```python
from build123d import *

# Parameters (mm, degrees)
BASE_FLANGE1_START             = -2
BASE_FLANGE1_DEPTH             = 2
EDGE_FLANGE1_STRIP_W           = 9.4732
EDGE_FLANGE1_STRIP_H           = 2
EDGE_FLANGE1_STRIP_CUT_DEPTH   = 254
EDGE_FLANGE1_STRIP_2_W         = 9.4732
EDGE_FLANGE1_STRIP_2_H         = 2
EDGE_FLANGE1_STRIP_CUT_2_DEPTH = 254
EDGE_FLANGE1_DEPTH             = 254
EDGE_FLANGE1_BEND_DEPTH        = 254
EDGE_FLANGE2_STRIP_W           = 9.4732
EDGE_FLANGE2_STRIP_H           = 2
EDGE_FLANGE2_STRIP_CUT_DEPTH   = 220
EDGE_FLANGE2_DEPTH             = 220
SKETCH15_R                     = 2
SKETCH15_R_2                   = 9.75
CUT_EXTRUDE1_DEPTH             = 178.482393493
SKETCH16_W                     = 25
SKETCH16_H                     = 7
SKETCH16_R                     = 2
CUT_EXTRUDE2_DEPTH             = 261.384331326


# Read off the part's stored shape, not the designer's step: Base-Flange1
# Sheet-metal steps are written as plain solids
with BuildPart() as part:
    # Base-Flange1 outline → Base-Flange1 (new body)
    with BuildSketch(Plane(origin=(0, 0, 0), x_dir=(1, 0, 0), z_dir=(0, 1, 0)).offset(BASE_FLANGE1_START)):
        Polygon((105, 126), (110, 126), (110, 130), (-110, 130), (-110, 126), (-105, 126), (-105, 124), (-110, 124), (-110, -130), (110, -130), (110, 124), (105, 124), align=None)
    extrude(amount=BASE_FLANGE1_DEPTH)

    # Edge-Flange1 strip (across the edge) → Edge-Flange1 strip cut (cut)
    with BuildSketch(Plane(origin=(-110, 0, -124), x_dir=(1, 0, 0), z_dir=(0, 0, 1))):
        with Locations((-2, -1)):
            Rectangle(EDGE_FLANGE1_STRIP_W, EDGE_FLANGE1_STRIP_H)
    extrude(amount=EDGE_FLANGE1_STRIP_CUT_DEPTH, mode=Mode.SUBTRACT)

    # Edge-Flange1 strip 2 (across the edge) → Edge-Flange1 strip cut 2 (cut)
    with BuildSketch(Plane(origin=(110, 0, 130), x_dir=(-1, 0, 0), z_dir=(0, 0, -1))):
        with Locations((-2, -1)):
            Rectangle(EDGE_FLANGE1_STRIP_2_W, EDGE_FLANGE1_STRIP_2_H)
    extrude(amount=EDGE_FLANGE1_STRIP_CUT_2_DEPTH, mode=Mode.SUBTRACT)

    # Edge-Flange1 section (across the edge) → Edge-Flange1 (add)
    with BuildSketch(Plane(origin=(-110, 0, -124), x_dir=(1, 0, 0), z_dir=(0, 0, 1))):
        with BuildLine():
            Line((0, 0.7366), (0, 50))
            Line((0, 50), (2, 50))
            Line((2, 50), (2, 0.7366))
            ThreePointArc((2, 0.7366), (2.215745145, 0.215745145), (2.7366, 0))
            Line((2.7366, 0), (2.7366, -2))
            ThreePointArc((2.7366, -2), (0.801531583, -1.198468417), (0, 0.7366))
        make_face()
    extrude(amount=EDGE_FLANGE1_DEPTH)

    # Edge-Flange1 section 2 (across the edge) → Edge-Flange1 bend (add)
    with BuildSketch(Plane(origin=(110, 0, 130), x_dir=(-1, 0, 0), z_dir=(0, 0, -1))):
        with BuildLine():
            Line((0, 0.7366), (0, 50))
            Line((0, 50), (2, 50))
            Line((2, 50), (2, 0.7366))
            ThreePointArc((2, 0.7366), (2.215745145, 0.215745145), (2.7366, 0))
            Line((2.7366, 0), (2.7366, -2))
            ThreePointArc((2.7366, -2), (0.801531583, -1.198468417), (0, 0.7366))
        make_face()
    extrude(amount=EDGE_FLANGE1_BEND_DEPTH)

    # Edge-Flange2 strip (across the edge) → Edge-Flange2 strip cut (cut)
    with BuildSketch(Plane(origin=(110, 0, -130), x_dir=(0, 0, 1), z_dir=(-1, 0, 0))):
        with Locations((-2, -1)):
            Rectangle(EDGE_FLANGE2_STRIP_W, EDGE_FLANGE2_STRIP_H)
    extrude(amount=EDGE_FLANGE2_STRIP_CUT_DEPTH, mode=Mode.SUBTRACT)

    # Edge-Flange2 section (across the edge) → Edge-Flange2 (add)
    with BuildSketch(Plane(origin=(110, 0, -130), x_dir=(0, 0, 1), z_dir=(-1, 0, 0))):
        with BuildLine():
            Line((0, 0.7366), (0, 3))
            Line((0, 3), (2, 3))
            Line((2, 3), (2, 0.7366))
            ThreePointArc((2, 0.7366), (2.215745145, 0.215745145), (2.7366, 0))
            Line((2.7366, 0), (2.7366, -2))
            ThreePointArc((2.7366, -2), (0.801531583, -1.198468417), (0, 0.7366))
        make_face()
    extrude(amount=EDGE_FLANGE2_DEPTH)

    # Sketch15 → Cut-Extrude1 (cut, through all)
    with BuildSketch(Plane(origin=(0, 0, 0), x_dir=(1, 0, 0), z_dir=(0, 1, 0))):
        Polygon((-85, -15), (-85, 105), (85, 105), (85, -15), (65, -45), (-65, -45), align=None)
        with Locations(Location((82, -107, 0), (0, 0, 270))):
            Circle(SKETCH15_R)
        with Locations(Location((67.5, -92.5, 0), (0, 0, 270))):
            Circle(SKETCH15_R)
        with Locations(Location((53, -107, 0), (0, 0, 270))):
            Circle(SKETCH15_R)
        with Locations(Location((67.5, -121.5, 0), (0, 0, 270))):
            Circle(SKETCH15_R)
        with Locations(Location((67.5, -107, 0), (0, 0, 270))):
            Circle(SKETCH15_R_2)
        with BuildLine():
            ThreePointArc((0, -85.5), (-10.5, -96), (0, -106.5))
            Line((0, -106.5), (0, -85.5))
        make_face()
        with BuildLine():
            Line((0, -85.5), (0, -106.5))
            ThreePointArc((0, -106.5), (7.424621202, -103.424621202), (10.5, -96))
            ThreePointArc((10.5, -96), (7.424621202, -88.575378798), (0, -85.5))
        make_face()
        with BuildLine():
            Line((0, -122), (0, -130))
            Line((0, -130), (65, -130))
            ThreePointArc((65, -130), (62.885553403, -129.850222745), (60.81333294, -129.403882079))
            Line((60.81333294, -129.403882079), (37.391782876, -122.596117921))
            ThreePointArc((37.391782876, -122.596117921), (35.319562413, -122.149777255), (33.205115817, -122))
            Line((33.205115817, -122), (0, -122))
        make_face()
        with BuildLine():
            Line((-65, -130), (0, -130))
            Line((0, -130), (0, -122))
            Line((0, -122), (-33.205115817, -122))
            ThreePointArc((-33.205115817, -122), (-35.319562413, -122.149777255), (-37.391782876, -122.596117921))
            Line((-37.391782876, -122.596117921), (-60.81333294, -129.403882079))
            ThreePointArc((-60.81333294, -129.403882079), (-62.885553403, -129.850222745), (-65, -130))
        make_face()
        with Locations(Location((16, -96, 0), (0, 0, 270))):
            Circle(SKETCH15_R)
        with Locations(Location((-16, -96, 0), (0, 0, 270))):
            Circle(SKETCH15_R)
        with Locations(Location((-67.5, -107, 0), (0, 0, 270))):
            Circle(SKETCH15_R_2)
        with Locations(Location((-53, -107, 0), (0, 0, 270))):
            Circle(SKETCH15_R)
        with Locations(Location((-67.5, -92.5, 0), (0, 0, 270))):
            Circle(SKETCH15_R)
        with Locations(Location((-67.5, -121.5, 0), (0, 0, 270))):
            Circle(SKETCH15_R)
        with Locations(Location((-82, -107, 0), (0, 0, 270))):
            Circle(SKETCH15_R)
        with Locations(Location((-90, -45, 0), (0, 0, 270))):
            Circle(SKETCH15_R)
        with Locations(Location((90, 115, 0), (0, 0, 90))):
            Circle(SKETCH15_R)
        with Locations(Location((90, -45, 0), (0, 0, 90))):
            Circle(SKETCH15_R)
        with Locations(Location((-90, 115, 0), (0, 0, 270))):
            Circle(SKETCH15_R)
    extrude(amount=-CUT_EXTRUDE1_DEPTH, mode=Mode.SUBTRACT)

    # Sketch16 → Cut-Extrude2 (cut, through all)
    with BuildSketch(Plane.ZY.offset(110)):
        with BuildLine():
            ThreePointArc((-124, 10.7366), (-122.535533906, 14.272133906), (-119, 15.7366))
            Line((-119, 15.7366), (53.501367481, 15.7366))
            ThreePointArc((53.501367481, 15.7366), (59.500667262, 17.736074884), (63.100877196, 22.934919573))
            Line((63.100877196, 22.934919573), (68.899122804, 42.801680427))
            ThreePointArc((68.899122804, 42.801680427), (72.499332738, 48.000525116), (78.498632519, 50))
            Line((78.498632519, 50), (-124, 50))
            Line((-124, 50), (-124, 10.7366))
        make_face()
        with Locations((38.5, 8.2366)):
            Rectangle(SKETCH16_W, SKETCH16_H)
        with Locations((3.5, 8.2366)):
            Rectangle(SKETCH16_W, SKETCH16_H)
        with Locations((-31.5, 8.2366)):
            Rectangle(SKETCH16_W, SKETCH16_H)
        with Locations((-66.5, 8.2366)):
            Rectangle(SKETCH16_W, SKETCH16_H)
        with Locations((-101.5, 8.2366)):
            Rectangle(SKETCH16_W, SKETCH16_H)
        with Locations(Location((86, 43, 0), (0, 0, 270))):
            Circle(SKETCH16_R)
        with Locations(Location((86, 23, 0), (0, 0, 270))):
            Circle(SKETCH16_R)
        with Locations(Location((119, 43, 0), (0, 0, 270))):
            Circle(SKETCH16_R)
        with Locations(Location((119, 23, 0), (0, 0, 270))):
            Circle(SKETCH16_R)
    extrude(amount=-CUT_EXTRUDE2_DEPTH, mode=Mode.SUBTRACT)


solid = part.part
```
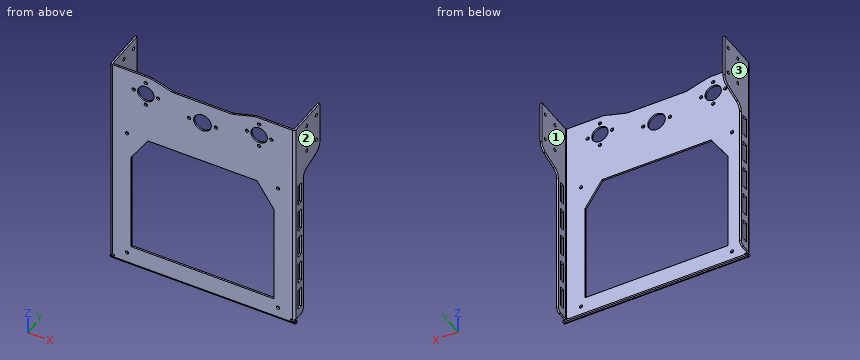
Geometry check sheet. Reference: the model listing, model coordinates, mm. Face numbers are marked on the shaded views. Coordinates: 2 decimals unless noted, no trailing zeros. Order: outer loops, then holes, each group sorted by start corner. A loop starts at its lowest first (then second) coordinate and runs counter-clockwise, first axis right, second up.
Item 1: Mould release check, pull along X, two halves, no side actions. Record for the marked faces 1, 2 and 3: released by +X, released by -X, zero draft, split by the parting line, or undercut.
Item 2: Scan lines: line 1 along Z through (x, y) = (-108.4, 23); line 2 along Z through (x, y) = (-109.3, 43); line 3 along X through (y, z) = (5, -17.5). Record each from-to range of solid material in increasing order.
Item 3: Section check A-A (z = -27). Enter the section's corners in (x, y), plus the area to 3 significant figures.
Item 4: Section check C-C (z = 20.5). Enter the section's corners in (x, y), plus the area to 3 significant figures.
Item 5: Section check B-B (y = 7.5). Count the separate pieces of the cut face and the enclosed holes in it, plus the area to 3 significant figures.
Item 6: Depth check by flat-ended pin: pin 1 (3.5 mm diameter, centred on x = 82, z = 107, fed in from -Y); pin 2 (1.6 mm diameter, centred on y = -1, z = -124.5, fed in from +X); pin 3 (2 mm diameter, centred on x = 19.5, y = -1, fed in from +Z); pin 4 (2 mm diameter, centred on x = -109, z = 9.5, fed in from -Y). Enter the tip coordinate at first touch or a pass-through.
Check sheet entries:
1. face 1: undercut
1. face 2: released by +X
1. face 3: released by -X
2. line 1: z = 63.12 to 84, 88 to 117, 121 to 130
2. line 2: z = 68.96 to 84, 88 to 117, 121 to 130
2. line 3: x = -110 to -108, 108 to 110
3. outline: (-110, 0.74) arc R2.74 ccw to (-107.26, -2) - (-85, -2) - (-85, 0) - (-107.26, 0) arc R0.74 cw to (-108, 0.74) - (-108, 4.74) - (-110, 4.74) - close; (-110, 11.74) - (-108, 11.74) - (-108, 15.74) - (-110, 15.74) - close; (85, -2) - (107.26, -2) arc R2.74 ccw to (110, 0.74) - (110, 4.74) - (108, 4.74) - (108, 0.74) arc R0.74 cw to (107.26, 0) - (85, 0) - close; (108, 11.74) - (110, 11.74) - (110, 15.74) - (108, 15.74) - close
3. area: 132 mm2
4. outline: (-110, 0.74) arc R2.74 ccw to (-107.26, -2) - (-81.33, -2) - (-81.33, 0) - (-107.26, 0) arc R0.74 cw to (-108, 0.74) - (-108, 15.74) - (-110, 15.74) - close; (81.33, -2) - (107.26, -2) arc R2.74 ccw to (110, 0.74) - (110, 15.74) - (108, 15.74) - (108, 0.74) arc R0.74 cw to (107.26, 0) - (81.33, 0) - close
4. area: 175 mm2
5. separate pieces: 12
5. enclosed holes: 0
5. area: 516 mm2
6. pin 1: passes through
6. pin 2: stops at x = 109.76
6. pin 3: stops at z = 122
6. pin 4: stops at y = -1.9
